The model under review builds one solid part; all positions refer to its coordinate system, in mm. Face numbers are marked on the shaded views. A direction names the side the tool comes from. Coordinates: 2 decimals unless noted, no trailing zeros. Loops run counter-clockwise (first coordinate to the right, second up) from the corner with the lowest first, then second, coordinate; pieces in that order, holes last. Notation, with made-up numbers: (10, -11.75) - (38, -11.75) arc R35 cw to (38, 25.25) - close; hole circle Ø1 at (45.25, -24.75). An arc over 180 degrees is marked (long way). One line per item, written item: value. Start each with the question number.
1. For the marked faces 1 and 2, list the 3-axis set-ups (+Z, -Z, +X, -X, +Y, -Y) from which the entire face can be reached by the end or side of a thin tool; tool diameter is ignored.
2. Insertion check: P1, Ø1, axis at y = -8.5, z = 5, coming from the +X side; P2, Ø3, axis at x = 7.5, y = -6.5, coming from the +Z side. Each pin has a flat end and moves straight along its axis. Give the tip position at first contact, or say it passes through.
3. To check wall thickness, follow line 1 (X direction, y = -2.25, z = 9); line 2 (Z direction, x = 10.5, y = -4.25). State the ranges of each line that lie inside material, in increasing order.
4. We need section B-B, the plane y = -6.5. Give the boundary of the cut face in (x, z).
5. We need section A-A, the plane x = 11.5. Give the boundary of the cut face in (y, z).
6. We need section C-C, the plane z = -2. Give the boundary of the cut face in (x, y), then the cut area to 3 significant figures.
from build123d import *

# Parameters (mm, degrees)
F0_W        = 10
F0_H        = 10
F1_DEPTH    = 10
F2_R        = 0.5
F3_T1_DEPTH = 11.5


# Not quite as in the source:
# - a fillet or chamfer that OpenCascade refuses, or shapes differently, is made with other operations: its cross-section is extruded or revolved along the edge and cut away or added


with BuildPart() as f1:
    # F0 (on Front) → F1 (new body)
    with BuildSketch(Plane.XZ):
        Polygon((5, 15), (-5, 15), (-5, -15), (5, -15), (5, -5), align=None)
        with Locations((10, -10)):
            Rectangle(F0_W, F0_H)
    extrude(amount=F1_DEPTH)

    # F2
    f2_edges = [f1.edges().sort_by_distance(p)[0] for p in [
        (0, -10, 15),
        (-5, -10, 0),
        (5, -10, -15),
        (15, -10, -10),
        (10, -10, -5),
        (5, -10, 5),
        (0, 0, 15),
        (-5, 0, 0),
        (5, 0, -15),
        (15, 0, -10),
        (10, 0, -5),
        (5, 0, 5),
    ]]
    fillet(f2_edges, radius=F2_R)

    # F3: fillet of radius 0.5 on 11 edges, made by hand

    # F3_s2 → F3_t1 (cut)
    with BuildSketch(Plane.XZ.offset(-0.75)):
        with BuildLine():
            ThreePointArc((-5, -14.5), (-4.8535533906, -14.8535533906), (-4.5, -15))
            Line((-4.5, -15), (-5, -15))
            Line((-5, -15), (-5, -14.5))
        make_face()
        with BuildLine():
            ThreePointArc((14.5, -15), (14.8535533906, -14.8535533906), (15, -14.5))
            Line((15, -14.5), (15, -15))
            Line((15, -15), (14.5, -15))
        make_face()
        with BuildLine():
            ThreePointArc((4.5, 15), (4.8535533906, 14.8535533906), (5, 14.5))
            Line((5, 14.5), (5, 15))
            Line((5, 15), (4.5, 15))
        make_face()
        with BuildLine():
            ThreePointArc((-4.5, 15), (-4.8535533906, 14.8535533906), (-5, 14.5))
            Line((-5, 14.5), (-5, 15))
            Line((-5, 15), (-4.5, 15))
        make_face()
        with BuildLine():
            ThreePointArc((14.5, -5), (14.8535533906, -5.1464466094), (15, -5.5))
            Line((15, -5.5), (15, -5))
            Line((15, -5), (14.5, -5))
        make_face()
    extrude(amount=F3_T1_DEPTH, mode=Mode.SUBTRACT)


solid = f1.part
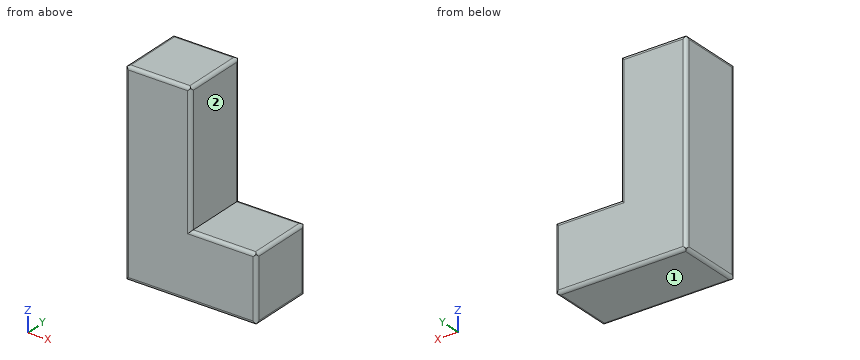
Findings below:
1. face 1: -Z, +X, -X, +Y, -Y
1. face 2: +Z, +X, +Y, -Y
2. P1: x = 5
2. P2: z = -5
3. line 1: -5 to 5
3. line 2: -15 to -5
4. outline: (-5, -14.5) arc R0.5 ccw to (-4.5, -15) - (14.5, -15) arc R0.5 ccw to (15, -14.5) - (15, -5.5) arc R0.5 ccw to (14.5, -5) - (5, -5) - (5, 14.5) arc R0.5 ccw to (4.5, 15) - (-4.5, 15) arc R0.5 ccw to (-5, 14.5) - close
5. outline: (-10, -14.5) arc R0.5 ccw to (-9.5, -15) - (-0.5, -15) arc R0.5 ccw to (0, -14.5) - (0, -5.5) arc R0.5 ccw to (-0.5, -5) - (-9.5, -5) arc R0.5 ccw to (-10, -5.5) - close
6. outline: (-5, -9.5) arc R0.5 ccw to (-4.5, -10) - (4.5, -10) arc R0.5 ccw to (5, -9.5) - (5, -0.5) arc R0.5 ccw to (4.5, 0) - (-4.5, 0) arc R0.5 ccw to (-5, -0.5) - close
6. area: 99.8 mm2
